Source: CAD feature listing. Evaluate the final solid. Frame: model axes, mm. Face numbers are marked on the shaded views. A direction names the side the tool comes from. Round coordinates to 2 decimals unless told otherwise and drop trailing zeros. Loops run counter-clockwise (first coordinate to the right, second up) from the corner with the lowest first, then second, coordinate; pieces in that order, holes last. Notation, with made-up numbers: (43, 58.5) -> (87, 58.5) arc R20 cw to (87, 90.5) -> close; hole circle Ø5 at (19, -9.5). An arc over 180 degrees is marked (long way). Write item = value, one per line.
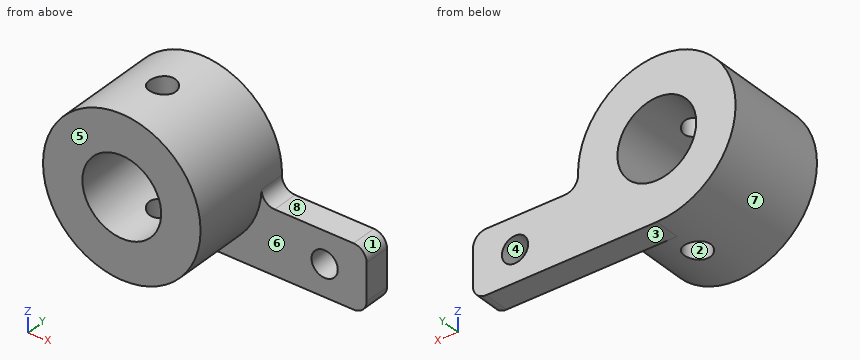
Autodesk Inventor part; units mm, degrees
ref_plane "YZ Plane" through (0, 0, 0) normal (1, 0, 0) x (0, 1, 0)
ref_plane "XZ Plane" through (0, 0, 0) normal (0, 1, 0) x (-1, 0, 0)
ref_plane "XY Plane" through (0, 0, 0) normal (0, 0, 1) x (1, 0, 0)
sketch "Sketch1" plane through (0, 0, 0) normal (0, 1, 0) x (-1, 0, 0)
  circle A0 centre (0, 0) radius 19.05
  circle A1 centre (0, 0) radius 9.525
  dimension "d0" = 38.1
  dimension "d1" = 19.05
extrude "Extrusion1" add sketch "Sketch1" along normal blind 25.4
sketch "Sketch2" plane through (0, 25.4, 0) normal (0, 1, 0) x (1, 0, 0)
  circle A0 centre (0, 0) radius 19.05
  line L0 (0, 19.05) -> (44.45, 19.05)
  line L1 (44.45, 19.05) -> (44.45, 3.81)
  line L2 (44.45, 3.81) -> (18.6651, 3.81)
  line L3 (44.45, 11.43) -> (15.24, 11.43)
  circle A1 centre (34.29, 11.43) radius 3.175
  dimension "d4" = 44.45
  dimension "d5" = 15.24
  dimension "d6" = 6.35
  dimension "d7" = 10.16
extrude "Extrusion2" add sketch "Sketch2" against normal blind 6.35 contours A0 L3 A1 L1 L2 | L0 L1 L3 A1 A0
fillet "Fillet1" radius 3.175 3 edges at (18.6651, 22.225, -3.81) (44.45, 22.225, -3.81) (44.45, 22.225, -19.05)
sketch "Sketch3" plane through (0, 19.05, -19.05) normal (0, 0, -1) x (-1, 0, 0)
  circle A0 centre (0, -6.35) radius 3.175
  line L0 (19.05, -19.05) -> (-19.05, -19.05)
  point P0 (0, -19.05)
  point P1 (0, -19.05)
  dimension "d11" = 12.7
  dimension "d12" = 6.35
extrude "Extrusion3" cut sketch "Sketch3" against normal through all
properties part number "ShaftGuide" material "Aluminum 6061"
1. Set-up query: the marked faces 5, 6, 7 and 8. Return all of +Z, -Z, +X, -X, +Y, -Y with unobstructed straight access to the full face (end or side cutting, diameter ignored); none if empty.
Evaluation:
face_5 = +Z, -Z, +X, -X, -Y
face_6 = -Z, +X, -Y
face_7 = -Y
face_8 = +Z, +X, +Y, -Y
2. Section query D-D (y = 23). Return the cut outline in (x, z) (3 decimals).
Evaluation:
outline = (0, -19.05) -> (41.275, -19.05) arc R3.175 ccw to (44.45, -15.875) -> (44.45, -6.985) arc R3.175 ccw to (41.275, -3.81) -> (22.216, -3.81) arc R3.175 cw to (19.042, -0.544) arc R19.05 ccw (long way) to start; hole circle Ø19.05 at (0, 0); hole circle Ø6.35 at (34.29, -11.43)
3. Contact query for flat-ended pins moving along their axis: pin 1 Ø2 at (y, z) = (11.5, 4) entering from +X; pin 2 Ø4 at (y, z) = (11.5, 2.5) entering from -X; pin 3 Ø5.5 at (x, z) = (23.5, -13) entering from -Y. Output: stop coordinate, or through.
Evaluation:
pin_1 = 18.81
pin_2 = -19.04
pin_3 = 19.05
4. Section query C-C (z = 3.5). Return the cut outline in (x, y), then the cut area to 3 significant figures.
Evaluation:
outline = (-18.73, 0) -> (-8.86, 0) -> (-8.86, 25.4) -> (-18.73, 25.4) -> close; (8.86, 0) -> (18.73, 0) -> (18.73, 25.4) -> (8.86, 25.4) -> close
area = 501 mm²
5. Line query: probe 1 along Z at (x, y) = (34.29, 20.5) (3 decimals); probe 2 along Y at (x, z) = (0, 13) (3 decimals); probe 3 along Z at (x, y) = (31, 22.5). Output: solid intervals per line, ascending. Write a range as from..to.
Evaluation:
probe_1 = -19.05..-14.605, -8.255..-3.81
probe_2 = 0..9.525, 15.875..25.4
probe_3 = -19.05..-3.81
6. Section query A-A (z = -11.43). Return the cut outline in (x, y) (3 decimals), then the cut area to 3 significant figures.
Evaluation:
outline = (-15.24, 0) -> (15.24, 0) -> (15.24, 19.05) -> (31.115, 19.05) -> (31.115, 25.4) -> (-15.24, 25.4) -> close; (37.465, 19.05) -> (44.45, 19.05) -> (44.45, 25.4) -> (37.465, 25.4) -> close; hole circle Ø6.35 at (0, 12.7)
area = 888 mm²
7. Section query B-B (x = 34.29). Return the cut outline in (y, z) (3 decimals).
Evaluation:
outline = (19.05, -19.05) -> (25.4, -19.05) -> (25.4, -14.605) -> (19.05, -14.605) -> close; (19.05, -8.255) -> (25.4, -8.255) -> (25.4, -3.81) -> (19.05, -3.81) -> close
8. Mould query, pull axis Z, two halves, no side actions, for the marked faces 1, 2, 3 and 4. Classes: released by +Z, released by -Z, zero draft, split by the parting line, or undercut.
Evaluation:
face_1 = released by +Z
face_2 = zero draft
face_3 = released by -Z
face_4 = undercut
